For this review, take the finished solid that the model builds, in its own axes (mm). A direction names the side the tool comes from. Give positions to 0.01 mm unless a question says otherwise; leave off trailing zeros. Loops run counter-clockwise (first coordinate to the right, second up) from the corner with the lowest first, then second, coordinate; pieces in that order, holes last. Notation, with made-up numbers: (46, 78.5) -> (89, 78.5) arc R21 ccw to (89, 113.5) -> close; hole circle Ø9 at (71, -5.75). An arc over 180 degrees is marked (long way). Write each question's results on one line, items separated by ' | '. Start each with the question number.
Autodesk Inventor part; units mm, degrees
ref_plane "YZ Plane" through (0, 0, 0) normal (1, 0, 0) x (0, 1, 0)
ref_plane "XZ Plane" through (0, 0, 0) normal (0, 1, 0) x (-1, 0, 0)
ref_plane "XY Plane" through (0, 0, 0) normal (0, 0, 1) x (1, 0, 0)
sketch "Sketch1" plane through (0, 0, 0) normal (0, 1, 0) x (-1, 0, 0)
  line L0 (86.9, 54.4) -> (-86.9, 54.4)
  line L1 (-86.9, 54.4) -> (-86.9, -54.4)
  line L2 (-86.9, -54.4) -> (86.9, -54.4)
  line L3 (86.9, -54.4) -> (86.9, 54.4)
  line L4 (86.9, 54.4) -> (-86.9, -54.4) construction
  line L5 (-86.9, 54.4) -> (86.9, -54.4) construction
  point P0 (0, 0)
  dimension "d0" = 108.8
  dimension "d1" = 173.8
extrude "Extrusion1" add sketch "Sketch1" along normal blind 4
sketch "Sketch2" plane through (86.9, 0, 54.4) normal (1, 0, 0) x (0, 0, -1)
  line L0 (39.4, 6.5316) -> (69.4, 6.5316)
  line L1 (69.4, 6.5316) -> (69.4, -6.5316)
  line L2 (69.4, -6.5316) -> (39.4, -6.5316)
  line L3 (39.4, -6.5316) -> (39.4, 6.5316)
  line L4 (39.4, 6.5316) -> (69.4, -6.5316) construction
  line L5 (69.4, 6.5316) -> (39.4, -6.5316) construction
  line L6 (69.4, 0) -> (79.4, 0)
  line L7 (79.4, 0) -> (79.4, -2)
  line L8 (79.4, -2) -> (69.4, -2)
  line L9 (69.4, -2) -> (69.4, 0)
  line L10 (39.4, 0) -> (29.4, 0)
  line L11 (29.4, 0) -> (29.4, -2)
  line L12 (29.4, -2) -> (39.4, -2)
  line L13 (39.4, -2) -> (39.4, 0)
  line L14 (69.4, -2) -> (79.4, -2)
  line L15 (79.4, -2) -> (79.4, -7)
  line L16 (79.4, -7) -> (69.4, -7)
  line L17 (69.4, -7) -> (69.4, -2)
  line L18 (39.4, -2) -> (29.4, -2)
  line L19 (29.4, -2) -> (29.4, -7)
  line L20 (29.4, -7) -> (39.4, -7)
  line L21 (39.4, -7) -> (39.4, -2)
  point P0 (54.4, 0)
  point P1 (69.4, -6.5316)
  dimension "d4" = 30
  dimension "d5" = 2
  dimension "d6" = 2
  dimension "d7" = 5
  dimension "d8" = 10
  dimension "d9" = 5
  dimension "d10" = 10
  dimension "d11" = 10
  dimension "d12" = 10
extrude "Extrusion2" add sketch "Sketch2" against normal blind 3 contours L3 L12 L11 L10 | L6 L7 L8 L1 | L3 L21 L20 L19 L12 | L8 L15 L16 L17 L1
sketch "Sketch3" plane through (86.9, 0, -54.4) normal (1, 0, 0) x (0, 0, -1)
  line L0 (-79.4, -2) -> (-69.4, -2)
  line L1 (-69.4, -7) -> (-69.4, -2)
  line L2 (-79.4, -7) -> (-69.4, -7)
  line L3 (-79.4, -2) -> (-79.4, -7)
  line L4 (-29.4, -2) -> (-39.4, -2)
  line L5 (-29.4, -2) -> (-29.4, -7)
  line L6 (-29.4, -7) -> (-39.4, -7)
  line L7 (-39.4, -7) -> (-39.4, -2)
  line L8 (-79.4, -7) -> (-69.4, -7)
  line L9 (-77.4, -2) -> (-71.4, -2)
  line L10 (-69.4, -4) -> (-69.4, -5)
  line L11 (-71.4, -7) -> (-77.4, -7)
  line L12 (-79.4, -5) -> (-79.4, -4)
  line L13 (-37.4, -2) -> (-31.4, -2)
  line L14 (-29.4, -4) -> (-29.4, -5)
  line L15 (-31.4, -7) -> (-37.4, -7)
  line L16 (-39.4, -5) -> (-39.4, -4)
  arc A0 (-37.4, -2) -> (-39.4, -4) centre (-37.4, -4) ccw
  arc A1 (-29.4, -4) -> (-31.4, -2) centre (-31.4, -4) ccw
  arc A2 (-31.4, -7) -> (-29.4, -5) centre (-31.4, -5) ccw
  arc A3 (-39.4, -5) -> (-37.4, -7) centre (-37.4, -5) ccw
  arc A4 (-77.4, -2) -> (-79.4, -4) centre (-77.4, -4) ccw
  arc A5 (-69.4, -4) -> (-71.4, -2) centre (-71.4, -4) ccw
  arc A6 (-71.4, -7) -> (-69.4, -5) centre (-71.4, -5) ccw
  arc A7 (-79.4, -5) -> (-77.4, -7) centre (-77.4, -5) ccw
  point P0 (-54.4, 0)
  dimension "d15" = 2
extrude "Extrusion3" add sketch "Sketch3" along normal blind 8 contours L0 A5 L1 A6 L2 A7 L3 A4 | A1 L5 A2 L6 A3 L7 A0 L4
sketch "Sketch4" plane through (94.9, 0, -54.4) normal (1, 0, 0) x (0, 0, -1)
  line L0 (-77.4, -7) -> (-71.4, -7)
  arc A0 (-71.4, -7) -> (-69.4, -5) centre (-71.4, -5) ccw
  line L1 (-69.4, -5) -> (-69.4, -4)
  arc A1 (-69.4, -4) -> (-71.4, -2) centre (-71.4, -4) ccw
  line L2 (-71.4, -2) -> (-77.4, -2)
  arc A2 (-77.4, -2) -> (-79.4, -4) centre (-77.4, -4) ccw
  line L3 (-79.4, -4) -> (-79.4, -5)
  arc A3 (-79.4, -5) -> (-77.4, -7) centre (-77.4, -5) ccw
  line L4 (-37.4, -7) -> (-31.4, -7)
  arc A4 (-31.4, -7) -> (-29.4, -5) centre (-31.4, -5) ccw
  line L5 (-29.4, -5) -> (-29.4, -4)
  arc A5 (-29.4, -4) -> (-31.4, -2) centre (-31.4, -4) ccw
  line L6 (-31.4, -2) -> (-37.4, -2)
  arc A6 (-37.4, -2) -> (-39.4, -4) centre (-37.4, -4) ccw
  line L7 (-39.4, -4) -> (-39.4, -5)
  arc A7 (-39.4, -5) -> (-37.4, -7) centre (-37.4, -5) ccw
  line L8 (-79.4, 0) -> (-79.4, -4)
  line L9 (-79.4, -2) -> (-69.4, -2)
  line L10 (-69.4, -2) -> (-69.4, -8.3081)
  line L11 (-69.4, -8.3081) -> (-79.4, -8.3081)
  line L12 (-79.4, -8.3081) -> (-79.4, -2)
  line L13 (-39.4, -7) -> (-39.4, 0)
  line L14 (-39.4, -2) -> (-29.4, -2)
  line L15 (-29.4, -2) -> (-29.4, -9.9458)
  line L16 (-29.4, -9.9458) -> (-39.4, -9.9458)
  line L17 (-39.4, -9.9458) -> (-39.4, -2)
  point P0 (-54.4, 0)
  point P1 (-29.4, -5)
extrude "Extrusion4" cut sketch "Sketch4" against normal through all contours L0 A0 L10 L11 L12 A3 | L4 A4 L15 L16 L17 L13 A7
fillet "Fillet1" radius 2 4 edges at (86.9, 2, 54.4) (86.9, 2, -54.4) (-86.9, 2, -54.4) (-86.9, 2, 54.4)
sketch "Sketch5" plane through (0, 4, 0) normal (0, 1, 0) x (1, 0, 0)
  circle A0 centre (0, 0) radius 17.5
  dimension "d21" = 35
extrude "Extrusion5" cut sketch "Sketch5" against normal blind 10
fillet "Fillet2" radius 1 2 edges at (-17.5, 0, 0) (-17.5, 4, 0)
properties part number "tapa de caja"
1. Machinability: for faces 4 (the flat face through (91, -2, -20)), 5 (the flat face through (87, -4.7, -15)), 6 (the flat face through (87, -4.7, 25)), 7 (the flat face through (83.9, -3, -20)), 8 (the flat face through (87, -4.7, -25)), which of the approach directions +Z, -Z, +X, -X, +Y, -Y give a long, thin tool a straight path to every point of the face, cutting with its end or side? Answer none if there is none.
2. We need section B-B (z = 0). Write out the cut boundary in (x, y).
3. We need section A-A (x = 0). Write out the cut boundary in (y, z).
4. We need section D-D (x = 81). Write out the cut boundary in (y, z), plus the area to 3 significant figures.
5. We need section C-C (z = -32). Write out the cut boundary in (x, y).
6. Wall thickness on L1, parallel to Z at x = 0, y = 2.3; L2, parallel to X at y = 1.7, z = 0; L3, parallel to X at y = 1.25, z = 9: over which ranges is each line inside the solid? List them lowest first.
7. Draft analysis for pull direction Z (two halves, no side actions). For faces 1 (the flat face through (21, 4, 1)), 2 (the flat face through (-1, 2, 54.4)), 3 (the flat face through (87, -4.2, 15)), state which applies: released by +Z, released by -Z, zero draft, split by the parting line, or undercut.
8. For pin 1 Ø4 at (x, y) = (89, -3.5) entering from +Z; pin 2 Ø3.5 at (y, z) = (-5, -20.5) entering from -X; pin 3 Ø1.5 at (x, y) = (91, -2) entering from -Z; pin 4 Ø21 at (x, z) = (0, 0) entering from +Y, all flat-tipped, find the tip position at first contact; note any pin that passes through.
Response:
1) face 4: +Z, -Z, +X, +Y | face 5: +X, -X, -Y | face 6: +Z, +X, -X, -Y | face 7: +Z, -Z, -X, -Y | face 8: -Z, +X, -X, -Y
2) outline: (-86.9, 0) -> (-18.5, 0) arc R1 ccw to (-17.5, 1) -> (-17.5, 3) arc R1 ccw to (-18.5, 4) -> (-86.9, 4) -> close; (17.5, 1) arc R1 ccw to (18.5, 0) -> (86.9, 0) -> (86.9, 4) -> (18.5, 4) arc R1 ccw to (17.5, 3) -> close
3) outline: (0, -54.4) -> (4, -54.4) -> (4, -18.5) arc R1 ccw to (3, -17.5) -> (1, -17.5) arc R1 ccw to (0, -18.5) -> close; (0, 18.5) arc R1 ccw to (1, 17.5) -> (3, 17.5) arc R1 ccw to (4, 18.5) -> (4, 54.4) -> (0, 54.4) -> close
4) outline: (0, -54.4) -> (4, -54.4) -> (4, 54.4) -> (0, 54.4) -> close | area: 435 mm2
5) outline: (-86.9, 0) -> (86.9, 0) -> (86.9, 4) -> (-86.9, 4) -> close
6) L1: z = -54.4 to -17.5, 17.5 to 54.4 | L2: x = -86.9 to -17.5, 17.5 to 86.9 | L3: x = -86.9 to -15.01, 15.01 to 86.9
7) face 1: zero draft | face 2: released by +Z | face 3: undercut
8) pin 1: stops at z = 25 | pin 2: stops at x = 83.9 | pin 3: stops at z = -24.56 | pin 4: passes through
